Study the drawing (mm; zero at the part's minimum x, y, z) and answer. A direction names the side the tool comes from. Round coordinates to 2 decimals unless told otherwise and drop trailing zeros. Write each loop counter-clockwise with the first axis right and the second up, starting at its lowest first coordinate (ties: lowest second). Pieces come first, ordered by that corner, then holes.
(1) Find the intervals of material crossed by probe 1 along Z at (x, y) = (3, 47); probe 2 along Z at (x, y) = (5.5, 22.5); probe 3 along Y at (x, z) = (2.2, 37), in increasing order.
(2) A cutting plane is placed at A-A, the plane z = 8.5. Give the vertices of the cut face in (x, y).
(3) The mould has two halves that part along Z. Classify the marked faces 1, 2 and 3: +Z half, -Z half, draft (parallel to the pull), parting line (faces both ways), or undercut.
(4) Each of these flat-tipped pins is pushed along its axis until it touches: pin 1 Ø2 at (y, z) = (21.5, 27) entering from -X; pin 2 Ø1.8 at (x, z) = (49, 8) entering from -Y; pin 3 Ø2.5 at (x, y) = (47.5, 42.6) entering from -Z; pin 4 Ø8 at (x, y) = (24.5, 7.5) entering from +Z. Where does it stop, or does it pass through?
(5) For the marked faces 4 and 5, determine the directions among +Z, -Z, +X, -X, +Y, -Y from which every point of the face is accessible in a straight line to the end or side of a thin tool.
(6) A cutting plane is placed at D-D, the plane x = 4.5. Give the vertices of the cut face in (y, z), and give its area (3 significant figures).
(7) A cutting plane is placed at B-B, the plane y = 23. Give the vertices of the cut face in (x, z).
(8) A cutting plane is placed at C-C, the plane z = 25. Give the vertices of the cut face in (x, y).
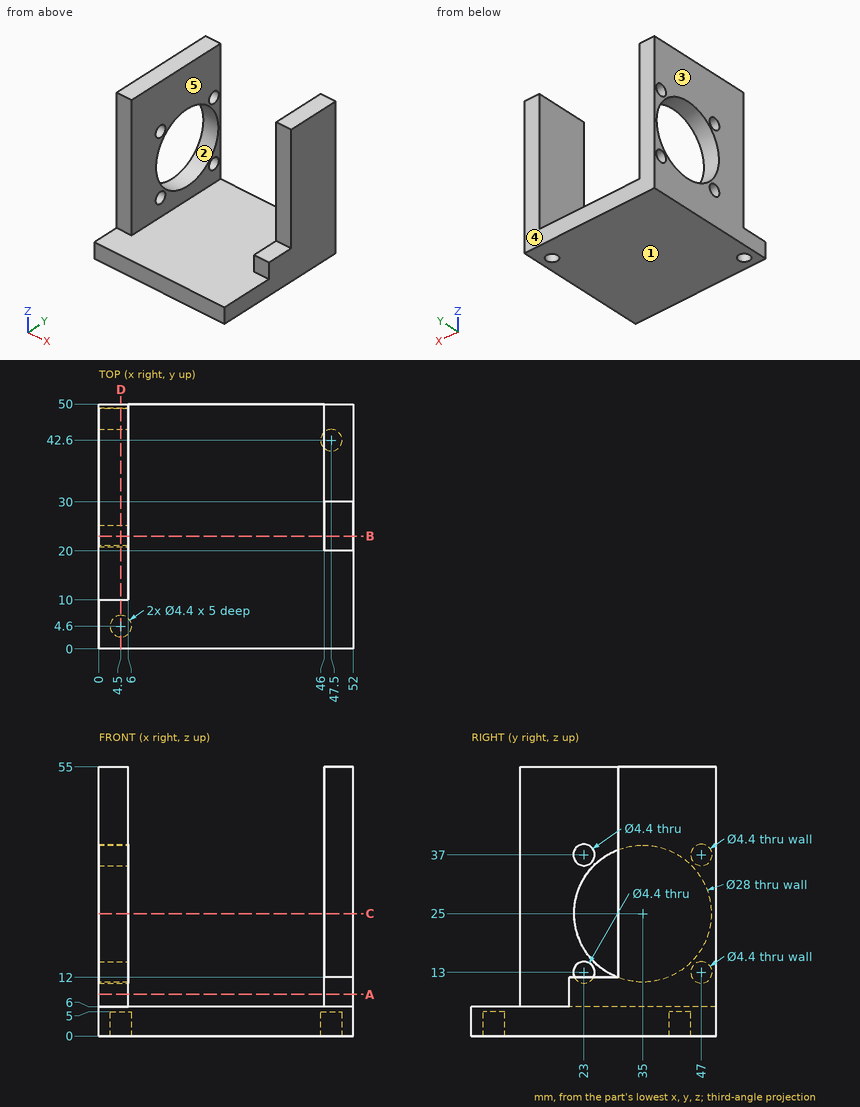
Solutions:
1. probe 1: z = 0 to 10.8, 15.2 to 17.79, 32.21 to 34.8, 39.2 to 55
1. probe 2: z = 0 to 10.86, 15.14 to 18.7, 31.3 to 34.86, 39.14 to 55
1. probe 3: y = 10 to 20.8, 25.2 to 27.79, 42.21 to 44.8, 49.2 to 50
2. outline: (0, 10) - (6, 10) - (6, 50) - (0, 50) - close; (46, 20) - (52, 20) - (52, 50) - (46, 50) - close
3. face 1: -Z half
3. face 2: undercut
3. face 3: draft
4. pin 1: stops at x = 0
4. pin 2: stops at y = 20
4. pin 3: stops at z = 5
4. pin 4: stops at z = 6
5. face 4: +Z, -Z, +X, -X, +Y
5. face 5: +Z, +Y, -Y
6. outline: (0, 0) - (2.4, 0) - (2.4, 5) - (6.8, 5) - (6.8, 0) - (50, 0) - (50, 55) - (10, 55) - (10, 6) - (0, 6) - close; hole circle Ø4.4 at (23, 13); hole circle Ø4.4 at (23, 37); hole circle Ø28 at (35, 25); hole circle Ø4.4 at (47, 13); hole circle Ø4.4 at (47, 37)
6. area: 1,560 mm2
7. outline: (0, 0) - (52, 0) - (52, 12) - (46, 12) - (46, 6) - (6, 6) - (6, 10.8) - (0, 10.8) - close; (0, 15.2) - (6, 15.2) - (6, 17.79) - (0, 17.79) - close; (0, 32.21) - (6, 32.21) - (6, 34.8) - (0, 34.8) - close; (0, 39.2) - (6, 39.2) - (6, 55) - (0, 55) - close
8. outline: (0, 10) - (6, 10) - (6, 21) - (0, 21) - close; (0, 49) - (6, 49) - (6, 50) - (0, 50) - close; (46, 30) - (52, 30) - (52, 50) - (46, 50) - close
